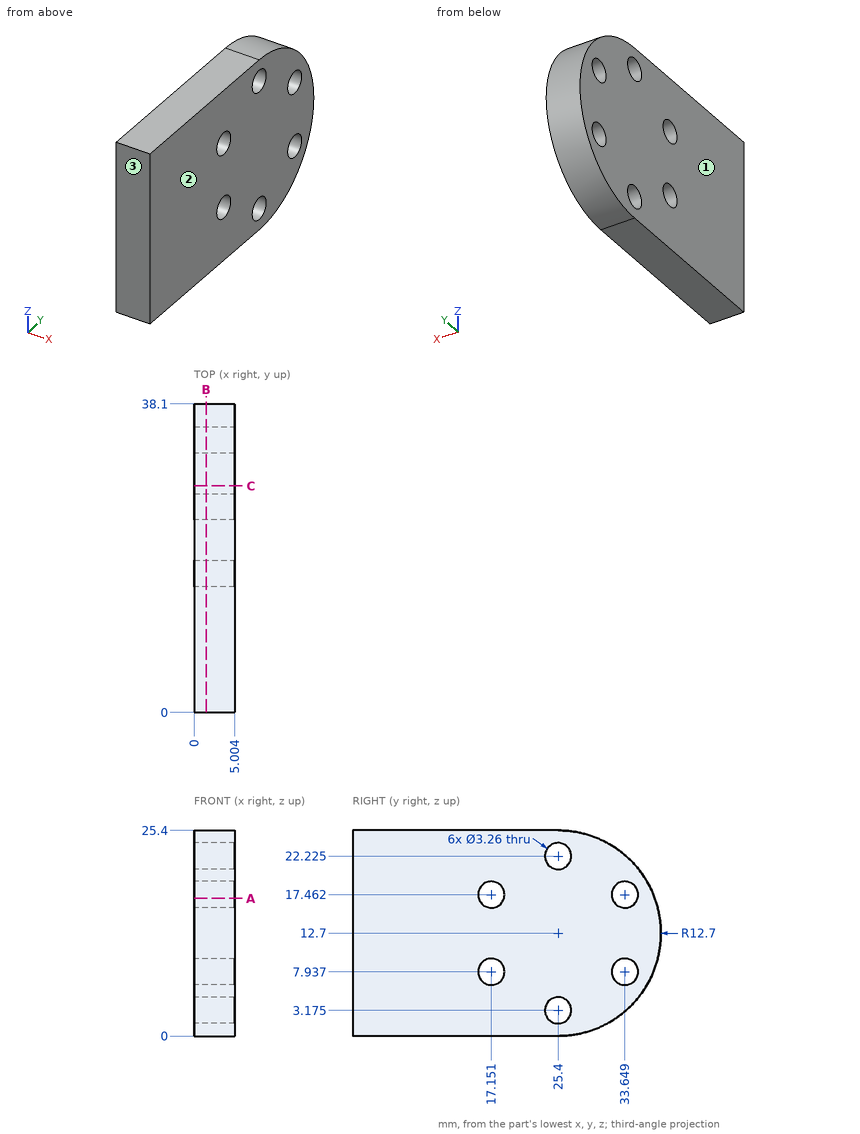
Geometry: see drawing. Coordinates: mm, zero at the bounding-box minimum. Give positions to 0.01 mm unless a question says otherwise; leave off trailing zeros. Order: outer loops, then holes, each group sorted by start corner. A loop starts at its lowest first (then second) coordinate and runs counter-clockwise, first axis right, second up. Notation, with made-up numbers: M 76,-18 L 91,-18 A18 cw 91,-14 Z; hole C 60,-20.5 d10. An arc over 180 degrees is marked long. Answer as a JSON object with one key per item and string values.
1. Cut plane C-C, the plane y = 28. Output: boundary loops of the cut face in (x, z), and give its area (3 significant figures).
Result sheet:
{"outline": "M 0,0.27 L 5,0.27 L 5,25.13 L 0,25.13 Z", "area": "124 mm²"}
2. Cut plane A-A, the plane z = 17. State how many separate pieces and enclosed holes the cut face has, and give its area (3 significant figures).
Result sheet:
{"separate pieces": "3", "enclosed holes": "0", "area": "156 mm²"}
3. Ray query, line 1 (Z direction, x = 2.5, y = 25.4) (1 decimal); line 2 (Z direction, x = 0.75, y = 26) (1 decimal); line 3 (Y direction, x = 3.45, z = 6.5) (1 decimal). Return the intervals inside material, ascending. Write a range as [from, to].
Result sheet:
{"line 1": "[0, 1.5], [4.8, 20.6], [23.9, 25.4]", "line 2": "[0, 1.7], [4.7, 20.7], [23.7, 25.4]", "line 3": "[0, 16.4], [17.9, 32.9], [34.4, 36.5]"}
4. First-contact query: P1, Ø3.5, axis at y = 33.65, z = 17.46, coming from the +X side; P2, Ø2.5, axis at y = 25.4, z = 22.225, coming from the +X side; P3, Ø3, axis at x = 2.5, z = 22, coming from the +Y side. Flat tips, straight axial feed; report the tip coordinate or a pass-through.
Result sheet:
{"P1": "x = 5", "P2": "through", "P3": "y = 35.42"}
5. Pull-direction query (X, two-part tool) for the marked faces 1, 2 and 3; classes: +X half, -X half, draft (parallel to the pull), parting line (faces both ways), or undercut.
Result sheet:
{"face 1": "-X half", "face 2": "+X half", "face 3": "draft"}
6. Cut plane B-B, the plane x = 1.5. Output: boundary loops of the cut face in (y, z) (1 decimal).
Result sheet:
{"outline": "M 0,0 L 25.4,0 A12.7 ccw 25.4,25.4 L 0,25.4 Z; hole C 17.2,7.9 d3.3; hole C 17.2,17.5 d3.3; hole C 25.4,3.2 d3.3; hole C 25.4,22.2 d3.3; hole C 33.6,7.9 d3.3; hole C 33.6,17.5 d3.3"}
